from build123d import *

# Parameters (mm, degrees)
F1_R     = 3
F2_DEPTH = 12
F3_COUNT = 10


# Not quite as in the source:
# - the dataset's text gives a spline's control points without its knots; the knots are read off the source's solid


with BuildPart() as f2:
    # F1 (on Top) → F2 (new body)
    with BuildSketch(Plane.XY):
        with BuildLine():
            add(Edge.make_bspline(
                [(1.1767889059, 18.3623301318), (1.6271784454, 17.7151013205), (2.818419618, 15.5665856482), (2.7289393763, 13.8155375104), (2.1532964325, 12.516122182)],
                knots=[0, 0, 0, 0, 0.4901902273, 1, 1, 1, 1], degree=3))
            ThreePointArc((1.1767889059, 18.3623301318), (0, 18.4), (-1.1767889059, 18.3623301318))
            add(Edge.make_bspline(
                [(-1.1767889059, 18.3623301318), (-1.6271784454, 17.7151013205), (-2.818419618, 15.5665856482), (-2.7289393763, 13.8155375104), (-2.1532964325, 12.516122182)],
                knots=[0, 0, 0, 0, 0.4901902273, 1, 1, 1, 1], degree=3))
            ThreePointArc((-2.1532964325, 12.516122182), (0, -12.7), (2.1532964325, 12.516122182))
        make_face()
        Circle(F1_R, mode=Mode.SUBTRACT)
    extrude(amount=F2_DEPTH)

    # F3: F2 ×10 about axis
    f3_axis = Axis((0, 0, 0), (0, 0, -1))


with BuildPart() as f2_1:
    add(f2.part)
    for i in range(1, F3_COUNT):
        add(f2.part.rotate(f3_axis, i * 360 / F3_COUNT))


solid = f2_1.part
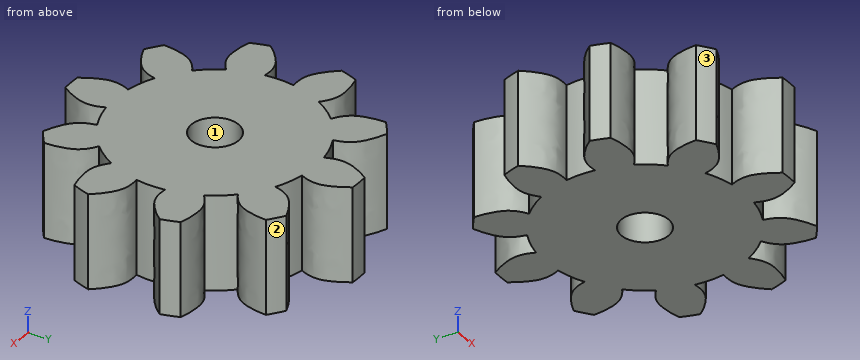
The listing builds one solid part. Answer for the finished solid, in the listing's coordinates (mm). Face numbers are marked on the shaded views. Coordinates: 2 decimals unless noted, no trailing zeros. Write each loop counter-clockwise with the first axis right and the second up, starting at its lowest first coordinate (ties: lowest second). Pieces come first, ordered by that corner, then holes. Notation, with made-up numbers: (6.25, 46.5) -> (54.25, 46.5) arc R16 cw to (54.25, 58.5) -> close; hole circle Ø11 at (65, -7.5). An arc over 180 degrees is marked (long way). One line per question, with ' | ' between items.
1. For a pull along X with two mould halves and no side action, classify the marked faces 1, 2 and 3 as released by +X, released by -X, zero draft, split by the parting line, or undercut.
Verdict:
face 1: undercut | face 2: released by +X | face 3: released by -X
2. Section A-A (x = 0) is taken. Determine the outline of the cut face in (y, z).
Verdict:
outline: (-18.4, 0) -> (-3, 0) -> (-3, 12) -> (-18.4, 12) -> close; (3, 0) -> (18.4, 0) -> (18.4, 12) -> (3, 12) -> close
3. Section B-B (y = 0) is taken. Determine the outline of the cut face in (x, z).
Verdict:
outline: (-12.7, 0) -> (-3, 0) -> (-3, 12) -> (-12.7, 12) -> close; (3, 0) -> (12.7, 0) -> (12.7, 12) -> (3, 12) -> close
4. Given pin 1 Ø1.5 at (x, z) = (6, 9.5) entering from +Y; pin 2 Ø4 at (y, z) = (-7.5, 6.5) entering from -X; pin 3 Ø6 at (y, z) = (0.5, 6) entering from +X; pin 4 Ø10 at (x, y) = (7.5, -6) entering from -Z, each flat-ended and moving along its own axis, determine where each tip first touches the part or whether it passes through.
Verdict:
pin 1: stops at y = 13.75 | pin 2: stops at x = -17.56 | pin 3: stops at x = 16.9 | pin 4: stops at z = 0
5. Straight lines are drawn through the part: line 1 (Y direction, x = 0, z = 4.25); line 2 (X direction, y = -6.5, z = 1); line 3 (Y direction, x = 9.5, z = 1.5). For each, find the intervals that lie inside material, in ascending order.
Verdict:
line 1: y = -18.4 to -3, 3 to 18.4 | line 2: x = -17.21 to -11.97, -10.91 to 10.91, 11.97 to 17.21 | line 3: y = -15.42 to -9.11, -8.43 to 8.43, 9.11 to 15.42
